Check sheet for the modelled part. Datum: model origin and axes. Units: mm. A direction names the side the tool comes from. Round coordinates to 2 decimals unless told otherwise and drop trailing zeros. Loops run counter-clockwise (first coordinate to the right, second up) from the corner with the lowest first, then second, coordinate; pieces in that order, holes last. Notation, with made-up numbers: (74.5, 40.5) -> (91.5, 40.5) arc R20 ccw to (91.5, 47.5) -> close; hole circle Ø3 at (80.25, -12). An arc over 180 degrees is marked (long way). One line per item, written item: value. Start each with the question number.
1. Cross-section at C-C on y = 3.5. Record the cut outline in (x, z).
2. Set-up check for faces 4 (the face through (1.653, 3.364, 0.042)), 5 (the face through (2, 8, 0)): record each of +Z, -Z, +X, -X, +Y, -Y from which the full face is reachable in a straight line by a thin tool's end or side.
3. Release check for a two-part mould opening along X. For faces 1 (the face through (2.481, 10.028, 1.526)), 2 (the face through (7, 7, 0)), 3 (the face through (2, 8, -3)) record: +X half, -X half, draft (parallel to the pull), parting line (faces both ways), or undercut.
4. Go/stop test with flat-tipped pins: pin 1 (3 mm diameter, centred on x = 5.5, z = -2.5, fed in from -Y); pin 2 (1.9 mm diameter, centred on x = 2, z = 0, fed in from +Y); pin 3 (1 mm diameter, centred on x = -1.5, y = 3, fed in from +Z). Record where each tip stops, or that it passes through.
5. Material ranges on L1, parallel to X at y = 9.35, z = 0; L2, parallel to X at y = 8.25, z = 1; L3, parallel to Y at x = 1.25, z = -0.5, recorded low to high.
6. Cross-section at B-B on y = 10.25. Record the cut outline in (x, z).
from build123d import *

# Parameters (mm, degrees)
BOSS_EXTRUDE1_DEPTH = 12
FILLET3_R           = 3
SKETCH2_R           = 1.6
CUT_EXTRUDE1_DEPTH  = 20
SKETCH4_R           = 1.6
CUT_EXTRUDE2_DEPTH  = 4


with BuildPart() as part:
    # Sketch1 → Boss-Extrude1 (new body)
    with BuildSketch(Plane(origin=(0, 0, 0), x_dir=(1, 0, 0), z_dir=(0, 1, 0))):
        with BuildLine():
            Line((0, 3), (4, 3))
            ThreePointArc((4, 3), (7, 0), (4, -3))
            Line((4, -3), (0, -3))
            ThreePointArc((0, -3), (-3, 0), (0, 3))
        make_face()
    extrude(amount=BOSS_EXTRUDE1_DEPTH)

    # Fillet3
    fillet3_edges = [part.edges().sort_by_distance(p)[0] for p in [
        (2, 0, -3),
        (7, 0, 0),
        (2, 0, 3),
        (-3, 0, 0),
    ]]
    fillet(fillet3_edges, radius=FILLET3_R - 0.0001)  # a hair under: the kernel refuses the full size

    # Sketch2 → Cut-Extrude1 (cut)
    with BuildSketch(Plane.XY.offset(3)):
        with Locations((2, 4.925974627)):
            Circle(SKETCH2_R)
    extrude(amount=-CUT_EXTRUDE1_DEPTH, mode=Mode.SUBTRACT)

    # Sketch4 → Cut-Extrude2 (cut)
    with BuildSketch(Plane(origin=(0, 12, 0), x_dir=(1, 0, 0), z_dir=(0, 1, 0))):
        with Locations(Location((2, 0, 0), (0, 0, 270))):
            Circle(SKETCH4_R)
    extrude(amount=-CUT_EXTRUDE2_DEPTH, mode=Mode.SUBTRACT)


solid = part.part
Taken from the geometry:
1. outline: (0, -3) -> (1.27, -3) -> (1.27, 3) -> (0, 3) arc R3 ccw to start; (2.73, -3) -> (4, -3) arc R3 ccw to (4, 3) -> (2.73, 3) -> close
2. face 4: +Z, -Z
2. face 5: +Y
3. face 1: undercut
3. face 2: +X half
3. face 3: draft
4. pin 1: stops at y = 0.35
4. pin 2: stops at y = 8
4. pin 3: stops at z = 2.83
5. L1: x = -3 to 0.4, 3.6 to 7
5. L2: x = -2.83 to 0.75, 3.25 to 6.83
5. L3: y = 0.04 to 3.51, 6.34 to 8
6. outline: (0, -3) -> (4, -3) arc R3 ccw to (4, 3) -> (0, 3) arc R3 ccw to start; hole circle Ø3.2 at (2, 0)
